Part model, mm, in its own coordinate system. A direction names the side the tool comes from. Give positions to 0.01 mm unless a question says otherwise; leave off trailing zeros. Write each loop counter-clockwise with the first axis right and the second up, starting at its lowest first coordinate (ties: lowest second). Pieces come first, ordered by that corner, then holes. Notation, with made-up numbers: M -5.5,4 L 1.5,4 A30 ccw 1.5,30 Z; hole C 78.5,19.5 d1. An arc over 180 degrees is marked long. Answer as CSV lines item,"result". Start each with the question number.
Item 1: Band-saw the part on C-C, the plane y = -35. List the corners of the cut face in (x, z), then the cut area to 3 significant figures.
Item 2: Band-saw the part on D-D, the plane z = 3.5. Count the separate pieces of the cut face and the enclosed holes in it, then the cut area to 3 significant figures.
Item 3: Pin check, flat tip, straight feed: pin 1 (8 mm diameter, centred on x = -25.2, y = 35.15, fed in from -Z). Stop position of the tip, or through.
Item 4: Wall check: L1, parallel to Y at x = 50.8, z = 2; L2, parallel to X at y = 7.5, z = 1.5; L3, parallel to Y at x = -25.5, z = 2.25. Give the ranges that are in metal, low to high. Write a range as from..to.
Item 5: 3-axis set-ups, long thin cutter, end or side, ignore diameter. For faces 4 (the cylindrical face through (8.027, 52.429, 3.131)), 5 (the flat face through (-63.5, -1, 3)): which of +Z, -Z, +X, -X, +Y, -Y reach the whole face in a straight line?
Item 6: Band-saw the part on B-B, the plane x = 50.8. List the corners of the cut face in (y, z).
Item 7: Band-saw the part on A-A, the plane y = -69.85. List the corners of the cut face in (x, z), then the cut area to 3 significant figures.
Item 8: Two-plate mould, pull along X, no slides. Class faces 1 (the cylindrical face through (-61.69, -80.64, 3.22)), 2 (the cylindrical face through (-8.03, 11.48, 3.13)), 3 (the cylindrical face through (61.59, 80.74, 3.22)): +X half, -X half, draft (parallel to the pull), parting line (faces both ways), or undercut.
from build123d import *

# Parameters (mm, degrees)
SKETCH1_W           = 127
SKETCH1_H           = 165.1
SKETCH1_R           = 3.3734375
SKETCH1_R_2         = 14.2875
SKETCH1_R_3         = 2.5527
BOSS_EXTRUDE1_DEPTH = 6.35
FILLET1_R           = 6.35


with BuildPart() as part:
    # Sketch1 → Boss-Extrude1 (new body)
    with BuildSketch(Plane.XY):
        Rectangle(SKETCH1_W, SKETCH1_H)
        with Locations((-50.8, 69.85)):
            Circle(SKETCH1_R, mode=Mode.SUBTRACT)
        with Locations((50.8, 69.85)):
            Circle(SKETCH1_R, mode=Mode.SUBTRACT)
        with Locations((50.8, -69.85)):
            Circle(SKETCH1_R, mode=Mode.SUBTRACT)
        with Locations((-50.8, -69.85)):
            Circle(SKETCH1_R, mode=Mode.SUBTRACT)
        with Locations((0, -31.952201006)):
            Circle(SKETCH1_R_2, mode=Mode.SUBTRACT)
        with Locations((-35.1409, 4.732361785)):
            Circle(SKETCH1_R_2, mode=Mode.SUBTRACT)
        with Locations((25.197543761, 28.751609125)):
            Circle(SKETCH1_R_3, mode=Mode.SUBTRACT)
        with Locations((-25.197543761, 35.152792887)):
            Circle(SKETCH1_R_3, mode=Mode.SUBTRACT)
        with BuildLine():
            Line((-7.534569408, 7.305159048), (-7.454878346, 7.932548946))
            ThreePointArc((-7.454878346, 7.932548946), (-8.049848215, 11.522345151), (-10.517966807, 14.196109643))
            ThreePointArc((-10.517966807, 14.196109643), (-20.473004306, 34.552681909), (-5.744824378, 51.773992023))
            ThreePointArc((-5.744824378, 51.773992023), (-2.686624737, 53.7458036), (-1.213076708, 57.072856673))
            Line((-1.213076708, 57.072856673), (-1.133385646, 57.700246571))
            ThreePointArc((-1.133385646, 57.700246571), (3.751093684, 61.483722294), (7.534569408, 56.599242964))
            Line((7.534569408, 56.599242964), (7.454878346, 55.971853066))
            ThreePointArc((7.454878346, 55.971853066), (8.049848215, 52.38205686), (10.517966807, 49.708292369))
            ThreePointArc((10.517966807, 49.708292369), (20.473004306, 29.351720103), (5.744824378, 12.130409989))
            ThreePointArc((5.744824378, 12.130409989), (2.686624737, 10.158598412), (1.213076708, 6.831545339))
            Line((1.213076708, 6.831545339), (1.133385646, 6.204155441))
            ThreePointArc((1.133385646, 6.204155441), (-3.751093684, 2.420679717), (-7.534569408, 7.305159048))
        make_face(mode=Mode.SUBTRACT)
    extrude(amount=BOSS_EXTRUDE1_DEPTH)

    # Fillet1
    fillet1_edges = [part.edges().sort_by_distance(p)[0] for p in [
        (63.5, -82.55, 3.175),
        (-63.5, -82.55, 3.175),
        (-63.5, 82.55, 3.175),
        (63.5, 82.55, 3.175),
    ]]
    fillet(fillet1_edges, radius=FILLET1_R)


solid = part.part
Output:
1,outline,"M -63.5,0 L -13.96,0 L -13.96,6.35 L -63.5,6.35 Z; M 13.96,0 L 63.5,0 L 63.5,6.35 L 13.96,6.35 Z"
1,area,"629 mm²"
2,separate pieces,"1"
2,enclosed holes,"9"
2,area,"18,000 mm²"
3,pin 1,"z = 0"
4,L1,"-82.55..-73.22, -66.48..66.48, 73.22..82.55"
4,L2,"-63.5..-49.16, -21.12..-7.51, 1.33..63.5"
4,L3,"-82.55..-5.81, 15.28..32.62, 37.69..82.55"
5,face 4,"+Z, -Z"
5,face 5,"+Z, -Z, -X, +Y, -Y"
6,outline,"M -82.55,0 L -73.22,0 L -73.22,6.35 L -82.55,6.35 Z; M -66.48,0 L 66.48,0 L 66.48,6.35 L -66.48,6.35 Z; M 73.22,0 L 82.55,0 L 82.55,6.35 L 73.22,6.35 Z"
7,outline,"M -63.5,0 L -54.17,0 L -54.17,6.35 L -63.5,6.35 Z; M -47.43,0 L 47.43,0 L 47.43,6.35 L -47.43,6.35 Z; M 54.17,0 L 63.5,0 L 63.5,6.35 L 54.17,6.35 Z"
7,area,"721 mm²"
8,face 1,"-X half"
8,face 2,"undercut"
8,face 3,"+X half"
